from build123d import *

# Parameters (mm, degrees)
F1_DEPTH = 127


with BuildPart() as f1:
    # F0 (on Front) → F1 (new body)
    with BuildSketch(Plane.XZ):
        with BuildLine():
            ThreePointArc((-130.556, 0), (-203.909349, 177.090651), (-381, 250.444))
            Line((-381, 250.444), (-381, 101.6))
            ThreePointArc((-381, 101.6), (-309.157951, 71.842049), (-279.4, 0))
            ThreePointArc((-279.4, 0), (-309.157951, -71.842049), (-381, -101.6))
            Line((-381, -101.6), (-381, -250.444))
            ThreePointArc((-381, -250.444), (-203.909349, -177.090651), (-130.556, 0))
        make_face()
        with BuildLine():
            Line((-381, 101.6), (-381, 250.444))
            ThreePointArc((-381, 250.444), (-631.444, 0), (-381, -250.444))
            Line((-381, -250.444), (-381, -101.6))
            ThreePointArc((-381, -101.6), (-482.6, 0), (-381, 101.6))
        make_face()
        with BuildLine():
            Line((381, 250.444), (-381, 250.444))
            ThreePointArc((-381, 250.444), (-203.909349, 177.090651), (-130.556, 0))
            ThreePointArc((-130.556, 0), (-203.909349, -177.090651), (-381, -250.444))
            Line((-381, -250.444), (381, -250.444))
            ThreePointArc((381, -250.444), (130.556, 0), (381, 250.444))
        make_face()
        with BuildLine():
            ThreePointArc((631.444, 0), (558.090651, 177.090651), (381, 250.444))
            Line((381, 250.444), (381, 101.6))
            ThreePointArc((381, 101.6), (452.842049, 71.842049), (482.6, 0))
            ThreePointArc((482.6, 0), (452.842049, -71.842049), (381, -101.6))
            Line((381, -101.6), (381, -250.444))
            ThreePointArc((381, -250.444), (558.090651, -177.090651), (631.444, 0))
        make_face()
        with BuildLine():
            Line((381, 101.6), (381, 250.444))
            ThreePointArc((381, 250.444), (130.556, 0), (381, -250.444))
            Line((381, -250.444), (381, -101.6))
            ThreePointArc((381, -101.6), (279.4, 0), (381, 101.6))
        make_face()
    extrude(amount=F1_DEPTH)


solid = f1.part
Input: part model. Units: mm. Frame: model coordinates. Round coordinates to 2 decimals unless told otherwise and drop trailing zeros. Order: outer loops, then holes, each group sorted by start corner. A loop starts at its lowest first (then second) coordinate and runs counter-clockwise, first axis right, second up. Notation, with made-up numbers: (79.25, -21) - (100.25, -21) arc R30 cw to (100.25, 14) - close; hole circle Ø2 at (45.25, 71.5). An arc over 180 degrees is marked (long way). Answer as a JSON object with one key per item and string values. Group by question number.
(1) Cut plane B-B (z = -36.5). Return loops of the section in (x, y), then the cut area to 3 significant figures.
(2) Pin query (flat end, axial travel): P1, Ø2, axis at x = -404.5, y = -72, coming from the -Z side. Return the tip coordinate at first contact, or that it passes through.
(3) Cut plane D-D (x = -308). Return loops of the section in (y, z).
(4) Cut plane C-C (x = 354). Return loops of the section in (y, z), then the cut area to 3 significant figures.
(5) Cut plane A-A (y = -49.5). Return loops of the section in (x, z), then the cut area to 3 significant figures.
(6) Material intervals for probe 1 along X at (y, z) = (-48, -6); probe 2 along X at (y, z) = (-27.5, -56); probe 3 along Z at (x, y) = (460, -32), sorted ascending. Write a range as from..to.
Here are the results:
{
 "1": {"outline": "(-628.77, -127) - (-475.82, -127) - (-475.82, 0) - (-628.77, 0) - close; (-286.18, -127) - (286.18, -127) - (286.18, 0) - (-286.18, 0) - close; (475.82, -127) - (628.77, -127) - (628.77, 0) - (475.82, 0) - close", "area": "112,000 mm^2"},
 "2": {"P1": "stops at z = -249.43"},
 "3": {"outline": "(-127, -250.44) - (0, -250.44) - (0, -70.67) - (-127, -70.67) - close; (-127, 70.67) - (0, 70.67) - (0, 250.44) - (-127, 250.44) - close"},
 "4": {"outline": "(-127, -250.44) - (0, -250.44) - (0, -97.95) - (-127, -97.95) - close; (-127, 97.95) - (0, 97.95) - (0, 250.44) - (-127, 250.44) - close", "area": "38,700 mm^2"},
 "5": {"outline": "(-381, -250.44) - (381, -250.44) arc R250.44 ccw to (631.44, 0) arc R250.44 ccw to (381, 250.44) - (-381, 250.44) arc R250.44 ccw to start; hole circle Ø203.2 at (-381, 0); hole circle Ø203.2 at (381, 0)", "area": "514,000 mm^2"},
 "6": {"probe 1": "x = -631.37..-482.42, -279.58..279.58, 482.42..631.37", "probe 2": "x = -625.1..-465.77, -296.23..296.23, 465.77..625.1", "probe 3": "z = -237.66..-63.89, 63.89..237.66"}
}
